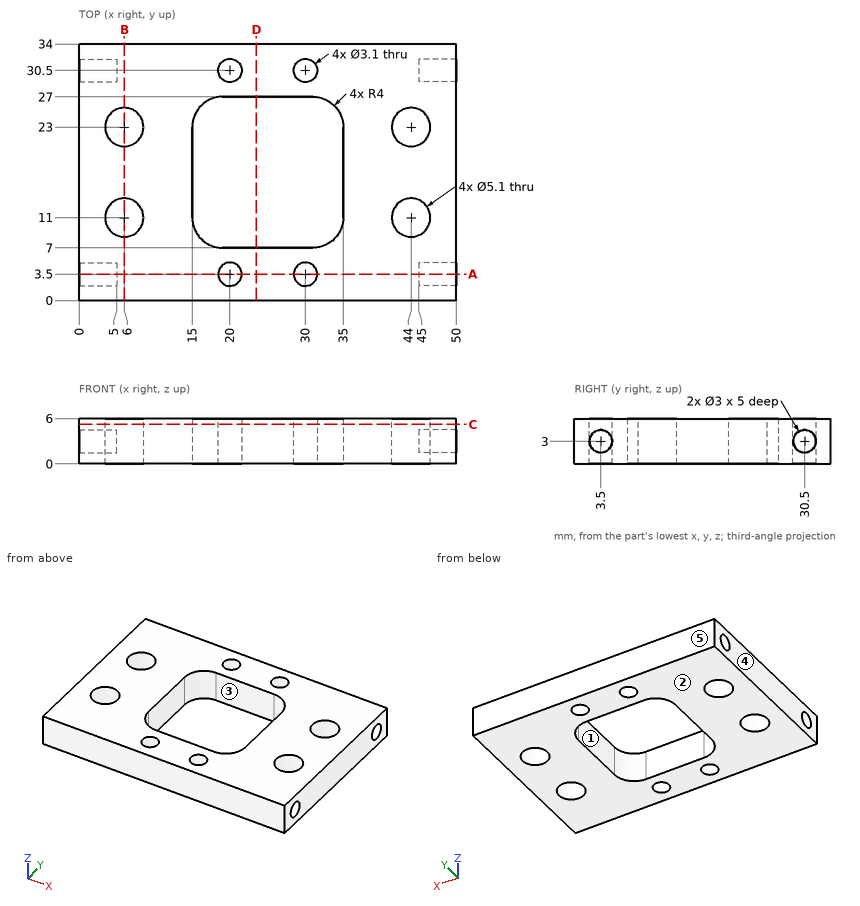
Design review of the part shown in the three views and the two pictorial views. Dimensions are in mm from the part's minimum x, y and z. A direction names the side the tool comes from. Round coordinates to 2 decimals unless told otherwise and drop trailing zeros. Loops run counter-clockwise (first coordinate to the right, second up) from the corner with the lowest first, then second, coordinate; pieces in that order, holes last. Notation, with made-up numbers: M -23.5,-16.75 L 29.5,-16.75 A22 cw 29.5,6.25 Z; hole C -25.75,-15.5 d1. An arc over 180 degrees is marked long. Answer as a JSON object with one key per item and string values.
Item 1: We need section C-C, the plane z = 5.25. State how many separate pieces and enclosed holes the cut face has, and give its area (3 significant figures).
Check sheet entries:
{"separate pieces": "1", "enclosed holes": "9", "area": "1,200 mm2"}
Item 2: Clearance check with flat-ended pins moving along their axes: P1, Ø0.9, axis at y = 30.5, z = 3.5, coming from the +X side; P2, Ø4, axis at x = 44, y = 11, coming from the +Z side; P3, Ø1.8, axis at y = 3.5, z = 3, coming from the -X side. State where each tip first meets the part, or that it passes through.
Check sheet entries:
{"P1": "x = 45", "P2": "through", "P3": "x = 5"}
Item 3: The part is to be moulded in two halves that separate along X. For the marked faces 3, 4 and 5, say which applies: +X half, -X half, draft (parallel to the pull), parting line (faces both ways), or undercut.
Check sheet entries:
{"face 3": "undercut", "face 4": "-X half", "face 5": "draft"}
Item 4: We need section B-B, the plane x = 6. State the section outline as (y, z) points, and give its area (3 significant figures).
Check sheet entries:
{"outline": "M 0,0 L 8.45,0 L 8.45,6 L 0,6 Z; M 13.55,0 L 20.45,0 L 20.45,6 L 13.55,6 Z; M 25.55,0 L 34,0 L 34,6 L 25.55,6 Z", "area": "143 mm2"}
Item 5: We need section D-D, the plane x = 23.5. State the section outline as (y, z) points, and give its area (3 significant figures).
Check sheet entries:
{"outline": "M 0,0 L 7,0 L 7,6 L 0,6 Z; M 27,0 L 34,0 L 34,6 L 27,6 Z", "area": "84.0 mm2"}
Item 6: For line 1 along X through (y, z) = (30.5, 3.45); line 2 along Y through (x, z) = (20, 4.45); line 3 along X through (y, z) = (19.5, 2.25), list the stretches that pass through material, from the lowest coordinate up.
Check sheet entries:
{"line 1": "5 to 18.45, 21.55 to 28.45, 31.55 to 45", "line 2": "0 to 1.95, 5.05 to 7, 27 to 28.95, 32.05 to 34", "line 3": "0 to 15, 35 to 50"}
Item 7: We need section A-A, the plane y = 3.5. State the section outline as (x, z) points.
Check sheet entries:
{"outline": "M 0,0 L 18.45,0 L 18.45,6 L 0,6 L 0,4.5 L 5,4.5 L 5,1.5 L 0,1.5 Z; M 21.55,0 L 28.45,0 L 28.45,6 L 21.55,6 Z; M 31.55,0 L 50,0 L 50,1.5 L 45,1.5 L 45,4.5 L 50,4.5 L 50,6 L 31.55,6 Z"}
Item 8: Tool access review of the marked faces 1 and 2: name each direction out of +Z, -Z, +X, -X, +Y, -Y from which nothing blocks a thin tool from reaching the whole face with its end or side.
Check sheet entries:
{"face 1": "+Z, -Z", "face 2": "-Z, +X, -X, +Y, -Y"}
